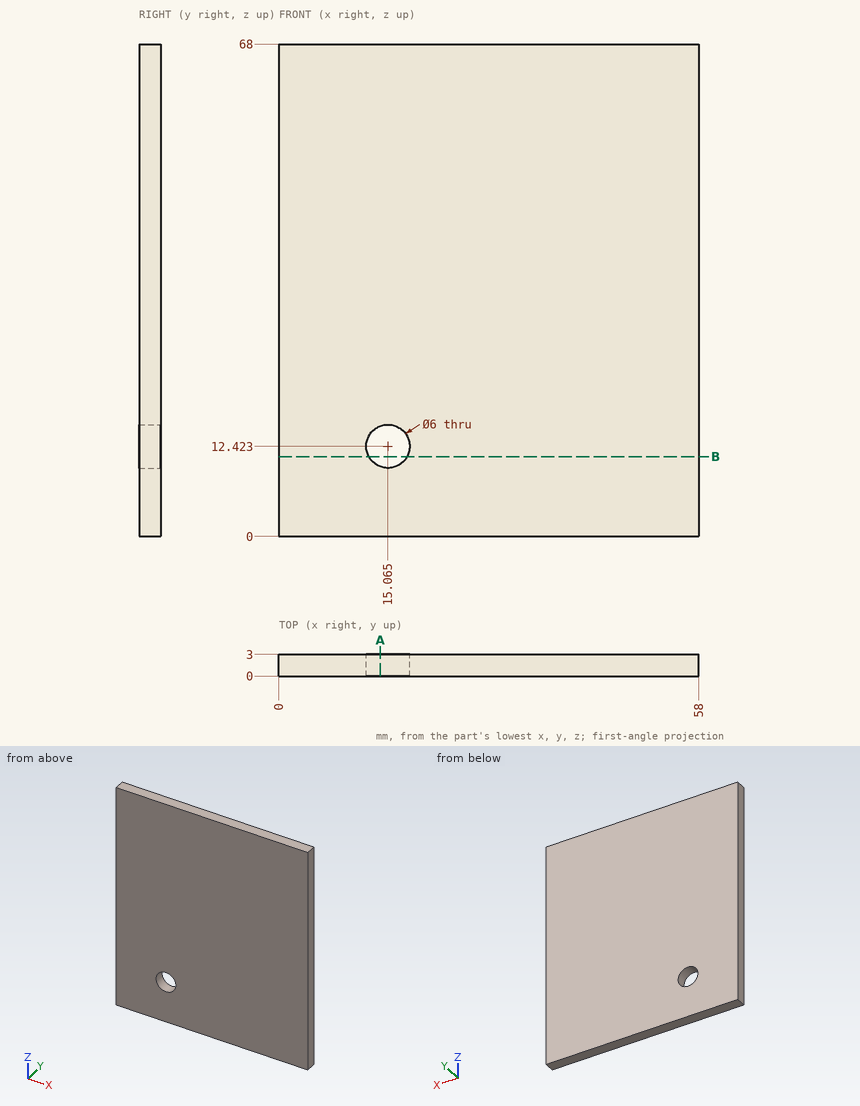
Design review of the part shown in the three views and the two pictorial views. Dimensions are in mm from the part's minimum x, y and z. Round coordinates to 2 decimals unless told otherwise and drop trailing zeros. Loops run counter-clockwise (first coordinate to the right, second up) from the corner with the lowest first, then second, coordinate; pieces in that order, holes last. Notation, with made-up numbers: (82.25, 77) - (124.25, 77) arc R32 ccw to (124.25, 113) - close; hole circle Ø4 at (30, -7). An arc over 180 degrees is marked (long way). Answer as CSV lines item,"result".
(1) Wall thickness on line 1 (X direction, y = 0.95, z = 14.5); line 2 (Z direction, x = 14, y = 1): over which ranges is each line inside the solid? List them lowest first.
Checked values:
line 1,"x = 0 to 12.9, 17.23 to 58"
line 2,"z = 0 to 9.62, 15.23 to 68"
(2) Consider section B-B on z = 11. Give the boundary of the cut face in (x, y).
Checked values:
outline,"(0, 0) - (12.42, 0) - (12.42, 3) - (0, 3) - close; (17.71, 0) - (58, 0) - (58, 3) - (17.71, 3) - close"
(3) Insertion check: P1, Ø5, axis at x = 15.06, z = 12.42, coming from the -Y side. The pin has a flat end and moves straight along its axis. Give the tip position at first contact, or say it passes through.
Checked values:
P1,"passes through"
(4) Consider section A-A on x = 14. Give the boundary of the cut face in (y, z).
Checked values:
outline,"(0, 0) - (3, 0) - (3, 9.62) - (0, 9.62) - close; (0, 15.23) - (3, 15.23) - (3, 68) - (0, 68) - close"
